Can you work these out from the model? Positions are in its coordinate system, mm. Face numbers are marked on the shaded views. A direction names the side the tool comes from. Round coordinates to 2 decimals unless told otherwise and drop trailing zeros. Loops run counter-clockwise (first coordinate to the right, second up) from the corner with the lowest first, then second, coordinate; pieces in that order, holes last. Notation, with made-up numbers: (7.5, 77) -> (37.5, 77) arc R30 ccw to (37.5, 113) -> close; hole circle Ø4 at (-34.5, 41). An arc over 180 degrees is marked (long way). Write item = value, one per line.
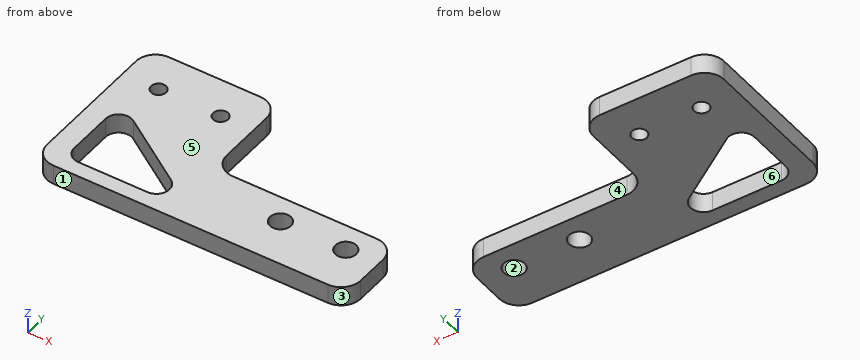
from build123d import *

# Parameters (mm, degrees)
SKETCH_1_W          = 48
SKETCH_1_H          = 67.5
SKETCH_1_R          = 1.6
SKETCH_1_R_2        = 1.15
EXTRUDE_1_DEPTH     = 3
SKETCH_3_W          = 28
SKETCH_3_H          = 56.5
CUT_EXTRUDE_1_DEPTH = 4
FILLET_1_R          = 3
SKETCH_5_W          = 37.363309984
SKETCH_5_H          = 43.840284148
CUT_EXTRUDE_2_DEPTH = 10
FILLET_2_R          = 3
CUT_EXTRUDE_3_DEPTH = 10
FILLET_3_R          = 2


with BuildPart() as part:
    # 草图1 → 凸台-拉伸1 (new body)
    with BuildSketch(Plane.XY):
        with Locations((24, 33.75)):
            Rectangle(SKETCH_1_W, SKETCH_1_H)
        with Locations((33, 7)):
            Circle(SKETCH_1_R, mode=Mode.SUBTRACT)
        with Locations((43, 7)):
            Circle(SKETCH_1_R, mode=Mode.SUBTRACT)
        with Locations((5.5, 20)):
            Circle(SKETCH_1_R_2, mode=Mode.SUBTRACT)
        with Locations((15, 20)):
            Circle(SKETCH_1_R_2, mode=Mode.SUBTRACT)
    extrude(amount=EXTRUDE_1_DEPTH)

    # 草图3 → 切除-拉伸1 (cut, through all)
    with BuildSketch(Plane.XY.offset(3)):
        with Locations((34, 39.25)):
            Rectangle(SKETCH_3_W, SKETCH_3_H)
    extrude(amount=-CUT_EXTRUDE_1_DEPTH, mode=Mode.SUBTRACT)

    # 圆角1
    fillet_1_edges = [part.edges().sort_by_distance(p)[0] for p in [
        (48, 11, 1.5),
        (20, 11, 1.5),
        (20, 67.5, 1.5),
        (0, 67.5, 1.5),
        (48, 0, 1.5),
        (0, 0, 1.5),
    ]]
    fillet(fillet_1_edges, radius=FILLET_1_R)

    # 草图5 → 切除-拉伸2 (cut)
    with BuildSketch(Plane.XY.offset(3)):
        with Locations((12.934999088, 47.920142074)):
            Rectangle(SKETCH_5_W, SKETCH_5_H)
    extrude(amount=-CUT_EXTRUDE_2_DEPTH, mode=Mode.SUBTRACT)

    # 圆角2
    fillet_2_edges = [part.edges().sort_by_distance(p)[0] for p in [
        (20, 26, 1.5),
        (0, 26, 1.5),
    ]]
    fillet(fillet_2_edges, radius=FILLET_2_R)

    # 草图6 → 切除-拉伸3 (cut)
    with BuildSketch(Plane.XY.offset(3)):
        Polygon((3.243199116, 15.127643762), (3.243199116, 2.334759345), (22.435417019, 2.334759345), align=None)
    extrude(amount=-CUT_EXTRUDE_3_DEPTH, mode=Mode.SUBTRACT)

    # 圆角3
    fillet_3_edges = [part.edges().sort_by_distance(p)[0] for p in [
        (3.243199116, 15.127643762, 1.5),
        (22.435417019, 2.334759345, 1.5),
        (3.243199116, 2.334759345, 1.5),
    ]]
    fillet(fillet_3_edges, radius=FILLET_3_R)


solid = part.part
1. Suppose I cut it at D-D, the plane y = 12. List the corners of the cut face in (x, z) for me.
Entries:
outline = (0, 0) -> (3.34, 0) -> (3.34, 3) -> (0, 3) -> close; (7.94, 0) -> (20.76, 0) -> (20.76, 3) -> (7.94, 3) -> close
2. For the marked faces 4, 5 and 6, which set-ups out of +Z, -Z, +X, -X, +Y, -Y let a thin tool reach every point of the face, with its end or its side?
Entries:
face_4 = +Z, -Z, +X, +Y
face_5 = +Z, +X, -X, +Y, -Y
face_6 = +Z, -Z
3. I need wall thicknesses on line 1 (Y direction, x = 33, z = 2.05); line 2 (Y direction, x = 6, z = 2.25); line 3 (Y direction, x = 39, z = 1.65). Which ranges of each line are inside material? Lowest first, please. Write a range as [from, to].
Entries:
line_1 = [0, 5.4], [8.6, 11]
line_2 = [0, 2.33], [13.24, 18.96], [21.04, 26]
line_3 = [0, 11]
4. We'd pull the mould along X, two halves only. Please class the marked faces 1, 2 and 3: released by +X, released by -X, zero draft, split by the parting line, or undercut.
Entries:
face_1 = zero draft
face_2 = undercut
face_3 = released by +X
5. Suppose I cut it at B-B, the plane y = 20. List the corners of the cut face in (x, z) for me, and give its area (3 significant figures).
Entries:
outline = (0, 0) -> (4.35, 0) -> (4.35, 3) -> (0, 3) -> close; (6.65, 0) -> (13.85, 0) -> (13.85, 3) -> (6.65, 3) -> close; (16.15, 0) -> (20, 0) -> (20, 3) -> (16.15, 3) -> close
area = 46.2 mm²
6. I'm going to push flat-ended pins straight in: pin 1 (1.5 mm diameter, centred on x = 33, z = 1.5, fed in from +Y); pin 2 (0.9 mm diameter, centred on y = 20.5, z = 1.5, fed in from +X). Where does each tip first touch, or does it pass through?
Entries:
pin_1 = 11
pin_2 = 20
7. Suppose I cut it at C-C, the plane z = 1.4. List the corners of the cut face in (x, y) for me.
Entries:
outline = (0, 3) arc R3 ccw to (3, 0) -> (45, 0) arc R3 ccw to (48, 3) -> (48, 8) arc R3 ccw to (45, 11) -> (23, 11) arc R3 cw to (20, 14) -> (20, 23) arc R3 ccw to (17, 26) -> (3, 26) arc R3 ccw to (0, 23) -> close; hole (3.24, 4.33) arc R2 ccw to (5.24, 2.33) -> (15.83, 2.33) arc R2 ccw to (16.94, 6) -> (6.35, 13.06) arc R2 ccw to (3.24, 11.39) -> close; hole circle Ø2.3 at (5.5, 20); hole circle Ø2.3 at (15, 20); hole circle Ø3.2 at (33, 7); hole circle Ø3.2 at (43, 7)
8. Suppose I cut it at A-A, the plane x = 33. List the corners of the cut face in (y, z) for me.
Entries:
outline = (0, 0) -> (5.4, 0) -> (5.4, 3) -> (0, 3) -> close; (8.6, 0) -> (11, 0) -> (11, 3) -> (8.6, 3) -> close
